Read the model definition and answer for the solid it produces. Units are mm, in the model's axes. A direction names the side the tool comes from. Round coordinates to 2 decimals unless told otherwise and drop trailing zeros. Write each loop counter-clockwise with the first axis right and the second up, starting at its lowest first coordinate (ties: lowest second). Pieces come first, ordered by that corner, then holes. Notation, with made-up numbers: (67, 39.5) - (89, 39.5) arc R17 cw to (89, 61.5) - close; hole circle Ø11 at (73, -32.75). An arc over 180 degrees is marked (long way). One line per item, written item: value. Start each with the question number.
(1) The mould has two halves that part along X. Classify faces 6 (the face through (40, 3, -3)), 7 (the face through (75, 3, -6)), 8 (the face through (114, 3, 10)): +X half, -X half, draft (parallel to the pull), parting line (faces both ways), or undercut.
(2) A cutting plane is placed at C-C, the plane z = 1.25. Determine the outline of the cut face in (x, y).
(3) For faces 1 (the face through (-3, 3, 15)), 2 (the face through (70, 3, -3)), 3 (the face through (111, 3, 5)), 4 (the face through (111, 3, 15)), 5 (the face through (15, 3, 0)), determine the directions among +Z, -Z, +X, -X, +Y, -Y from which every point of the face is accessible in a straight line to the end or side of a thin tool.
(4) Find the intervals of material crossed by L1, parallel to X at y = 3, z = -0.5; L2, parallel to X at y = 4, z = 11; L3, parallel to X at y = 2.75, z = 14.25, in increasing order.
(5) Flat-ended cylindrical pins translate along their axes: pin 1 Ø2 at (x, y) = (87, 1.5) entering from -Z; pin 2 Ø1.8 at (x, y) = (-3.5, 2.5) entering from +Z; pin 3 Ø2 at (y, z) = (4.5, -2) entering from +X. Find the tip coordinate at first contact, or state that the pin passes through.
(6) A cutting plane is placed at A-A, the plane z = 9. Determine the outline of the cut face in (x, y), plus the area to 3 significant figures.
(7) A cutting plane is placed at B-B, the plane x = 54. Determine the outline of the cut face in (y, z), plus the area to 3 significant figures.
from build123d import *

# Parameters (mm, degrees)
BOSS_EXTRUDE1_DEPTH = 6
FILLET1_R           = 5


with BuildPart() as part:
    # Sketch1 → Boss-Extrude1 (new body)
    with BuildSketch(Plane(origin=(0, 0, 0), x_dir=(1, 0, 0), z_dir=(0, 1, 0))):
        with BuildLine():
            Line((0, 0), (30, 0))
            Line((30, 0), (30, 6))
            Line((30, 6), (40, 6))
            Line((40, 6), (40, 0))
            Line((40, 0), (70, 0))
            Line((70, 0), (70, 6))
            Line((70, 6), (80, 6))
            Line((80, 6), (80, 0))
            Line((80, 0), (108, 0))
            Line((108, 0), (108, -5))
            Line((108, -5), (114, -5))
            Line((114, -5), (114, -15))
            Line((114, -15), (108, -15))
            Line((108, -15), (108, -20))
            ThreePointArc((108, -20), (90, -8), (72, -20))
            ThreePointArc((72, -20), (54, -8), (36, -20))
            ThreePointArc((36, -20), (18, -8), (0, -20))
            Line((0, -20), (0, -15))
            Line((0, -15), (-6, -15))
            Line((-6, -15), (-6, -5))
            Line((-6, -5), (0, -5))
            Line((0, -5), (0, 0))
        make_face()
    extrude(amount=BOSS_EXTRUDE1_DEPTH)

    # Fillet1
    fillet1_edges = [part.edges().sort_by_distance(p)[0] for p in [
        (72, 3, 20),
        (36, 3, 20),
    ]]
    fillet(fillet1_edges, radius=FILLET1_R)


solid = part.part
Here are the results:
1. face 6: undercut
1. face 7: draft
1. face 8: +X half
2. outline: (0, 0) - (108, 0) - (108, 6) - (0, 6) - close
3. face 1: +Z, -X, +Y, -Y
3. face 2: -Z, +Y, -Y
3. face 3: -Z, +X, +Y, -Y
3. face 4: +Z, +X, +Y, -Y
3. face 5: -Z, -X, +Y, -Y
4. L1: 30 to 40, 70 to 80
4. L2: -6 to 7.61, 28.39 to 43.61, 64.39 to 79.61, 100.39 to 114
4. L3: -6 to 3.69, 32.31 to 39.69, 68.31 to 75.69, 104.31 to 114
5. pin 1: z = 0
5. pin 2: z = 15
5. pin 3: x = 80
6. outline: (-6, 0) - (11.84, 0) - (11.84, 6) - (-6, 6) - close; (24.16, 0) - (47.84, 0) - (47.84, 6) - (24.16, 6) - close; (60.16, 0) - (83.84, 0) - (83.84, 6) - (60.16, 6) - close; (96.16, 0) - (114, 0) - (114, 6) - (96.16, 6) - close
6. area: 498 mm²
7. outline: (0, 0) - (6, 0) - (6, 8) - (0, 8) - close
7. area: 48.0 mm²
